```python
from build123d import *

# Parameters (mm, degrees)
F0_W     = 152.4
F0_H     = 31.75
F0_R     = 7.9375
F1_DEPTH = 3.175
F2_R     = 5.08


with BuildPart() as f1:
    # F0 (on Front) → F1 (new body, symmetric)
    with BuildSketch(Plane.XZ):
        with Locations((2.297985, 0)):
            Rectangle(F0_W, F0_H)
        with Locations((-58.027015, 0)):
            Circle(F0_R, mode=Mode.SUBTRACT)
    extrude(amount=F1_DEPTH, both=True)

    # F2
    f2_edges = [f1.edges().sort_by_distance(p)[0] for p in [
        (-73.902015, 0, 15.875),
        (-73.902015, 0, -15.875),
    ]]
    fillet(f2_edges, radius=F2_R)


solid = f1.part
```
Verification items for the finished model (mm, model axes). Coordinates: 2 decimals unless noted, no trailing zeros. Write each loop counter-clockwise with the first axis right and the second up, starting at its lowest first coordinate (ties: lowest second). Pieces come first, ordered by that corner, then holes. Notation, with made-up numbers: M 1.5,23.25 L 19.5,23.25 A17 cw 19.5,51.25 Z; hole C 54,34.25 d3. An arc over 180 degrees is marked long. Answer as a JSON object with one key per item and string values. Group by question number.
(1) Material ranges on line 1 (Z direction, x = -58.5, y = 1.5) (3 decimals); line 2 (X direction, y = 0, z = -1.5); line 3 (Z direction, x = -53.5, y = 2) (3 decimals), recorded low to high.
(2) Cross-section at C-C, the plane z = 6. Record the cut outline in (x, y) (3 decimals), and give its area (3 significant figures).
(3) Release check for a two-part mould opening along Z. For faces 1 (the face through (-72.5, 0, -14.3)), 2 (the face through (4, 0, 15.875)), 3 (the face through (-65.957, 0.044, 0.349)), 4 (the face through (1, -3.175, 0)) record: +Z half, -Z half, draft (parallel to the pull), parting line (faces both ways), or undercut.
(4) Cross-section at B-B, the plane y = 1.5. Record the cut outline in (x, z) (1 decimal).
(5) Cross-section at A-A, the plane z = 0. Record the cut outline in (x, y) (3 decimals), and give its area (3 significant figures).
(6) Gauge pin test, flat end, axial feed: pin 1 (14.5 mm diameter, centred on x = -58.03, z = 0, fed in from +Y). Record the tip position at first contact, or that the pin passes through.
Reply:
{
 "1": {"line 1": "-15.875 to -7.923, 7.923 to 15.875", "line 2": "-73.9 to -65.82, -50.23 to 78.5", "line 3": "-15.875 to -6.52, 6.52 to 15.875"},
 "2": {"outline": "M -73.902,-3.175 L -63.224,-3.175 L -63.224,3.175 L -73.902,3.175 Z; M -52.83,-3.175 L 78.498,-3.175 L 78.498,3.175 L -52.83,3.175 Z", "area": "902 mm²"},
 "3": {"face 1": "-Z half", "face 2": "+Z half", "face 3": "undercut", "face 4": "draft"},
 "4": {"outline": "M -73.9,-10.8 A5.1 ccw -68.8,-15.9 L 78.5,-15.9 L 78.5,15.9 L -68.8,15.9 A5.1 ccw -73.9,10.8 Z; hole C -58,0 d15.9"},
 "5": {"outline": "M -73.902,-3.175 L -65.965,-3.175 L -65.965,3.175 L -73.902,3.175 Z; M -50.09,-3.175 L 78.498,-3.175 L 78.498,3.175 L -50.09,3.175 Z", "area": "867 mm²"},
 "6": {"pin 1": "through"}
}
